```python
from build123d import *

# Parameters (mm, degrees)
RESSALTO_EXTRUS_O1_DEPTH   = 80
ESPELHAR2_COPY_1_DEPTH     = 80
ESBO_O2_R                  = 1.25
CORTE_EXTRUS_O1_DEPTH      = 1
CORTE_EXTRUS_O1_DEPTH_BACK = 161


with BuildPart() as part:
    # Esboço1 → Ressalto-extrusão1 (new body, symmetric)
    with BuildSketch(Plane.XY):
        Polygon((0, 2.35), (-0.825, 2.35), (-0.825, 2.95), (-2.9, 3.5), (-2.9, 6), (-1.6, 6), (-1.6, 7.5), (-4.4, 7.5), (-4.4, 5.460660172), (-6.439339828, 7.5), (-7.5, 7.5), (-7.5, 6.439339828), (-5.460660172, 4.4), (-7.5, 4.4), (-7.5, 1.6), (-6, 1.6), (-6, 2.9), (-3.5, 2.9), (-2.95, 0.825), (-2.35, 0.825), (-2.35, 0), (0, 0), align=None)
    ressalto_extrus_o1 = extrude(amount=RESSALTO_EXTRUS_O1_DEPTH, both=True)

    # Espelhar1: Ressalto-extrusão1 across plane
    add(ressalto_extrus_o1.mirror(Plane.ZX))

    # Espelhar2: Ressalto-extrusão1 across plane
    add(ressalto_extrus_o1.mirror(Plane(origin=(0, 0, 0), x_dir=(0, 0, 1), z_dir=(1, 0, 0))))

    # Espelhar2 copy 1 sketch → Espelhar2 copy 1 (add, symmetric)
    with BuildSketch(Plane(origin=(0, 0, 0), x_dir=(-1, 0, 0), z_dir=(0, 0, 1))):
        Polygon((0, 2.35), (-0.825, 2.35), (-0.825, 2.95), (-2.9, 3.5), (-2.9, 6), (-1.6, 6), (-1.6, 7.5), (-4.4, 7.5), (-4.4, 5.460660172), (-6.439339828, 7.5), (-7.5, 7.5), (-7.5, 6.439339828), (-5.460660172, 4.4), (-7.5, 4.4), (-7.5, 1.6), (-6, 1.6), (-6, 2.9), (-3.5, 2.9), (-2.95, 0.825), (-2.35, 0.825), (-2.35, 0), (0, 0), align=None)
    extrude(amount=ESPELHAR2_COPY_1_DEPTH, both=True)

    # Esboço2 → Corte-extrusão1 (cut, two sides)
    with BuildSketch(Plane.XY.offset(80)) as corte_extrus_o1_sk:
        Circle(ESBO_O2_R)
    extrude(amount=CORTE_EXTRUS_O1_DEPTH, mode=Mode.SUBTRACT)
    extrude(corte_extrus_o1_sk.sketch, amount=-CORTE_EXTRUS_O1_DEPTH_BACK, mode=Mode.SUBTRACT)


solid = part.part
```
Geometry check sheet. Reference: the model listing, model coordinates, mm. A direction names the side the tool comes from. Round coordinates to 2 decimals unless told otherwise and drop trailing zeros. Write item = value, one per line.
Q1. Set-up check for faces 1 (the flat face through (-3, -7.5, 1)), 2 (the flat face through (-5, 2.9, 1)): record each of +Z, -Z, +X, -X, +Y, -Y from which the full face is reachable in a straight line by a thin tool's end or side.
Answer block:
face_1 = +Z, -Z, +X, -X, -Y
face_2 = +Z, -Z
Q2. Depth check by flat-ended pin: pin 1 Ø0.8 at (x, z) = (-4.5, -0.5) entering from -Y; pin 2 Ø0.6 at (y, z) = (-6, -25) entering from +X; pin 3 Ø1.8 at (x, z) = (-0.5, -20.5) entering from +Y; pin 4 Ø3 at (y, z) = (0, -2.5) entering from -X. Enter the tip coordinate at first touch or a pass-through.
Answer block:
pin_1 = -7.5
pin_2 = 7.36
pin_3 = 3.1
pin_4 = -3.13
Q3. Scan lines: line 1 (X direction, y = 3.75, z = 6); line 2 (Y direction, x = 2, z = -70); line 3 (Y direction, x = -2.75, z = 59.5) (3 decimals). Record each from-to range of solid material in increasing order.
Answer block:
line_1 = -7.5 to -2.9, 2.9 to 7.5
line_2 = -7.5 to -6, -3.26 to 3.26, 6 to 7.5
line_3 = -7.5 to -6, -3.46 to -0.825, 0.825 to 3.46, 6 to 7.5
Q4. Release check for a two-part mould opening along Y. For faces 3 (the flat face through (5, -2.9, 1)), 4 (the flat face through (3, 7.5, 1)), 5 (the flat face through (0, -2, 80)) record: released by +Y, released by -Y, zero draft, split by the parting line, or undercut.
Answer block:
face_3 = undercut
face_4 = released by +Y
face_5 = zero draft
